Source: CAD feature listing. Evaluate the final solid. Frame: model axes, mm. A direction names the side the tool comes from. Give positions to 0.01 mm unless a question says otherwise; leave off trailing zeros. Order: outer loops, then holes, each group sorted by start corner. A loop starts at its lowest first (then second) coordinate and runs counter-clockwise, first axis right, second up.
from build123d import *

# Parameters (mm, degrees)
F0_W      = 100.33
F0_H      = 71.12
F0_W_2    = 90.17
F0_H_2    = 60.96
F1_DEPTH  = 5.08
F2_W      = 100.33
F2_H      = 71.12
F3_DEPTH  = 5.08
F0_R      = 1.375
F4_DEPTH  = 25.4
F5_R      = 3.1
F5_R_2    = 1.375
F6_DEPTH  = 3.556
F7_DEPTH  = 37.592
F8_W      = 13.716
F8_H      = 3.556
F9_DEPTH  = 5.08
F10_W     = 10.668
F10_H     = 5.715
F10_W_2   = 17.78
F10_H_2   = 9.144
F10_W_3   = 9.398
F10_H_3   = 8.89
F11_DEPTH = 5.08
F12_W     = 53.8226
F12_H     = 18.161
F13_DEPTH = 5.08
F14_R     = 1.905
F15_DEPTH = 71.121
F17_DEPTH = 71.121
F19_DEPTH = 5.08


with BuildPart() as f1:
    # F0 (on Top) → F1 (new body)
    with BuildSketch(Plane.XY):
        with Locations((42.545, 27.94)):
            Rectangle(F0_W, F0_H)
        with Locations((42.545, 27.94)):
            Rectangle(F0_W_2, F0_H_2, mode=Mode.SUBTRACT)
    extrude(amount=-F1_DEPTH)

    # F2 (on face) → F3 (join)
    with BuildSketch(Plane(origin=(0, 0, -5.08), x_dir=(1, 0, 0), z_dir=(0, 0, -1))):
        with Locations((42.545, -27.94)):
            Rectangle(F2_W, F2_H)
    extrude(amount=F3_DEPTH)

    # F0 (on Top) → F4 (cut)
    with BuildSketch(Plane.XY):
        with Locations((3.5, 52.38)):
            Circle(F0_R)
        with Locations((61.5, 52.38)):
            Circle(F0_R)
        with Locations((61.5, 3.5)):
            Circle(F0_R)
        with Locations((3.5, 3.5)):
            Circle(F0_R)
    extrude(amount=-F4_DEPTH, mode=Mode.SUBTRACT)

    # F5 (on face) → F6 (join)
    with BuildSketch(Plane.XY.offset(-5.08)):
        with Locations((3.5, 52.38)):
            Circle(F5_R)
        with Locations((3.5, 52.38)):
            Circle(F5_R_2, mode=Mode.SUBTRACT)
        with Locations((61.5, 52.38)):
            Circle(F5_R)
        with Locations((61.5, 52.38)):
            Circle(F5_R_2, mode=Mode.SUBTRACT)
        with Locations((61.5, 3.5)):
            Circle(F5_R)
        with Locations((61.5, 3.5)):
            Circle(F5_R_2, mode=Mode.SUBTRACT)
        with Locations((3.5, 3.5)):
            Circle(F5_R)
        with Locations((3.5, 3.5)):
            Circle(F5_R_2, mode=Mode.SUBTRACT)
    extrude(amount=F6_DEPTH)

    # F0 (on Top) → F7 (join)
    with BuildSketch(Plane.XY):
        with Locations((42.545, 27.94)):
            Rectangle(F0_W, F0_H)
        with Locations((42.545, 27.94)):
            Rectangle(F0_W_2, F0_H_2, mode=Mode.SUBTRACT)
    extrude(amount=F7_DEPTH)

    # F8 (on face) → F9 (cut, through all)
    with BuildSketch(Plane(origin=(-7.62, 0, 0), x_dir=(0, -1, 0), z_dir=(-1, 0, 0))):
        with Locations((-27.94, -2.032)):
            Rectangle(F8_W, F8_H)
    extrude(amount=-F9_DEPTH, mode=Mode.SUBTRACT)

    # F10 (on face) → F11 (cut, through all)
    with BuildSketch(Plane.XZ.offset(7.62)):
        with Locations((10.922, 1.5875)):
            Rectangle(F10_W, F10_H)
        with Locations((31.75, 3.302)):
            Rectangle(F10_W_2, F10_H_2)
        with Locations((53.594, 3.175)):
            Rectangle(F10_W_3, F10_H_3)
    extrude(amount=-F11_DEPTH, mode=Mode.SUBTRACT)

    # F12 (on face) → F13 (cut, through all)
    with BuildSketch(Plane.YZ.offset(92.71)):
        with Locations((28.8163, 7.8105)):
            Rectangle(F12_W, F12_H)
    extrude(amount=-F13_DEPTH, mode=Mode.SUBTRACT)

    # F14 (on face) → F15 (cut, through all)
    with BuildSketch(Plane.XZ.offset(7.62)):
        with Locations((31.9024, 19.304)):
            Circle(F14_R)
    extrude(amount=-F15_DEPTH, mode=Mode.SUBTRACT)

    # F16 (on face) → F17 (cut, through all)
    with BuildSketch(Plane.XZ.offset(7.62)):
        with BuildLine():
            Line((66.58, -5.08), (66.58, -10.16))
            Line((66.58, -10.16), (92.71, -10.16))
            Line((92.71, -10.16), (92.71, 37.592))
            Line((92.71, 37.592), (-7.62, 37.592))
            Line((-7.62, 37.592), (-7.62, -10.16))
            Line((-7.62, -10.16), (-2.54, -10.16))
            Line((-2.54, -10.16), (-2.54, -5.08))
            Line((-2.54, -5.08), (13.97, -5.08))
            ThreePointArc((13.97, -5.08), (16.664077, -3.964077), (17.78, -1.27))
            Line((17.78, -1.27), (17.78, 9.144))
            ThreePointArc((17.78, 9.144), (18.895923, 11.838077), (21.59, 12.954))
            Line((21.59, 12.954), (23.0124, 12.954))
            ThreePointArc((23.0124, 12.954), (25.706477, 14.069923), (26.8224, 16.764))
            Line((26.8224, 16.764), (26.8224, 20.574))
            ThreePointArc((26.8224, 20.574), (27.938323, 23.268077), (30.6324, 24.384))
            Line((30.6324, 24.384), (33.1724, 24.384))
            ThreePointArc((33.1724, 24.384), (35.866477, 23.268077), (36.9824, 20.574))
            Line((36.9824, 20.574), (36.9824, 16.764))
            ThreePointArc((36.9824, 16.764), (38.098323, 14.069923), (40.7924, 12.954))
            Line((40.7924, 12.954), (41.91, 12.954))
            ThreePointArc((41.91, 12.954), (44.604077, 11.838077), (45.72, 9.144))
            Line((45.72, 9.144), (45.72, -1.27))
            ThreePointArc((45.72, -1.27), (46.835923, -3.964077), (49.53, -5.08))
            Line((49.53, -5.08), (66.58, -5.08))
        make_face()
    extrude(amount=-F17_DEPTH, mode=Mode.SUBTRACT)

    # F18 (on face) → F19 (cut, through all)
    with BuildSketch(Plane.XY.offset(-5.08)):
        with BuildLine():
            Line((56.42, 10.16), (57.69, 10.16))
            ThreePointArc((57.69, 10.16), (59.486051, 10.903949), (60.23, 12.7))
            Line((60.23, 12.7), (60.23, 43.18))
            ThreePointArc((60.23, 43.18), (59.486051, 44.976051), (57.69, 45.72))
            Line((57.69, 45.72), (56.42, 45.72))
            ThreePointArc((56.42, 45.72), (54.623949, 46.463949), (53.88, 48.26))
            Line((53.88, 48.26), (53.88, 49.53))
            ThreePointArc((53.88, 49.53), (53.136051, 51.326051), (51.34, 52.07))
            Line((51.34, 52.07), (12.7, 52.07))
            ThreePointArc((12.7, 52.07), (10.903949, 51.326051), (10.16, 49.53))
            Line((10.16, 49.53), (10.16, 48.26))
            ThreePointArc((10.16, 48.26), (9.416051, 46.463949), (7.62, 45.72))
            Line((7.62, 45.72), (6.35, 45.72))
            ThreePointArc((6.35, 45.72), (4.553949, 44.976051), (3.81, 43.18))
            Line((3.81, 43.18), (3.81, 12.7))
            ThreePointArc((3.81, 12.7), (4.553949, 10.903949), (6.35, 10.16))
            Line((6.35, 10.16), (7.62, 10.16))
            ThreePointArc((7.62, 10.16), (9.416051, 9.416051), (10.16, 7.62))
            Line((10.16, 7.62), (10.16, 6.35))
            ThreePointArc((10.16, 6.35), (10.903949, 4.553949), (12.7, 3.81))
            Line((12.7, 3.81), (51.34, 3.81))
            ThreePointArc((51.34, 3.81), (53.136051, 4.553949), (53.88, 6.35))
            Line((53.88, 6.35), (53.88, 7.62))
            ThreePointArc((53.88, 7.62), (54.623949, 9.416051), (56.42, 10.16))
        make_face()
    extrude(amount=-F19_DEPTH, mode=Mode.SUBTRACT)


solid = f1.part
(1) Pin query (flat end, axial travel): pin 1 Ø4 at (y, z) = (-4, 2) entering from -X; pin 2 Ø3 at (x, y) = (61.5, 52.38) entering from +Z; pin 3 Ø3 at (y, z) = (-4.5, 18.5) entering from +X. Return the tip coordinate at first contact, or that it passes through.
(2) Section B-B, the plane z = 12. Return loops of the section in (x, y), plus the area to 3 significant figures.
(3) Section C-C, the plane y = 20. Return loops of the section in (x, z), plus the area to 3 significant figures.
(4) Draft query along Y for faces 1 (the cylindrical face through (16.634, 60.924, -3.994)), 2 (the flat face through (34, -7.62, -2)), 3 (the flat face through (32, 3.81, -8)), 4 (the cylindrical face through (9.396, 9.436, -7.584)). Return one class per face: +Y half, -Y half, draft (parallel to the pull), parting line (faces both ways), or undercut.
(5) Section D-D, the plane x = 16.5. Return loops of the section in (y, z).
(6) Section A-A, the plane x = 61.5. Return loops of the section in (y, z) (3 decimals).
(7) Access query for faces 5 (the flat face through (1, 27, -5.08)), 6 (the flat face through (32, -5, 7.874)), 7 (the flat face through (17.78, 61, 4)), 8 (the flat face through (45.72, 61, 4)). Directions: +Z, -Z, +X, -X, +Y, -Y. A direction counts if a zero-diameter tool reaches every point of the face in a straight line with its end or side. Return the directions, or none.
(8) Line query: line 1 along X through (y, z) = (13, -6); line 2 along Y through (x, z) = (41, 0.5); line 3 along X through (y, z) = (3, -7). Output: solid intervals per line, ascending.
Checks:
1. pin 1: stops at x = 17.78
1. pin 2: stops at z = -5.08
1. pin 3: stops at x = 36.98
2. outline: (19.07, -7.62) - (44.43, -7.62) - (44.43, -2.54) - (19.07, -2.54) - close; (19.07, 58.42) - (44.43, 58.42) - (44.43, 63.5) - (19.07, 63.5) - close
2. area: 258 mm2
3. outline: (-2.54, -10.16) - (3.81, -10.16) - (3.81, -5.08) - (-2.54, -5.08) - close; (60.23, -10.16) - (66.58, -10.16) - (66.58, -5.08) - (60.23, -5.08) - close
3. area: 64.5 mm2
4. face 1: draft
4. face 2: -Y half
4. face 3: undercut
4. face 4: undercut
5. outline: (-7.62, -10.16) - (3.81, -10.16) - (3.81, -5.08) - (-2.54, -5.08) - (-2.54, -4.12) - (-7.62, -4.12) - close; (52.07, -10.16) - (63.5, -10.16) - (63.5, -4.12) - (58.42, -4.12) - (58.42, -5.08) - (52.07, -5.08) - close
6. outline: (-7.62, -10.16) - (2.125, -10.16) - (2.125, -5.08) - (-7.62, -5.08) - close; (4.875, -10.16) - (51.005, -10.16) - (51.005, -5.08) - (4.875, -5.08) - close; (53.755, -10.16) - (63.5, -10.16) - (63.5, -5.08) - (53.755, -5.08) - close
7. face 5: +Z
7. face 6: -Y
7. face 7: +Z, -X, +Y, -Y
7. face 8: +Z, +X, +Y, -Y
8. line 1: x = -2.54 to 3.81, 60.23 to 66.58
8. line 2: y = -7.62 to -2.54, 58.42 to 63.5
8. line 3: x = -2.54 to 2.22, 4.78 to 60.22, 62.78 to 66.58
